Part print with two shaded views. Sizes in mm from the minimum x, y, z corner. A direction names the side the tool comes from. Give positions to 0.01 mm unless a question says otherwise; leave off trailing zeros. Loops run counter-clockwise (first coordinate to the right, second up) from the corner with the lowest first, then second, coordinate; pieces in that order, holes last. Notation, with made-up numbers: M 33.25,-31.5 L 90.25,-31.5 A38 cw 90.25,7.5 Z; hole C 0.5,68.25 d11. An arc over 180 degrees is marked long. Answer in a Markdown table with one row per item.
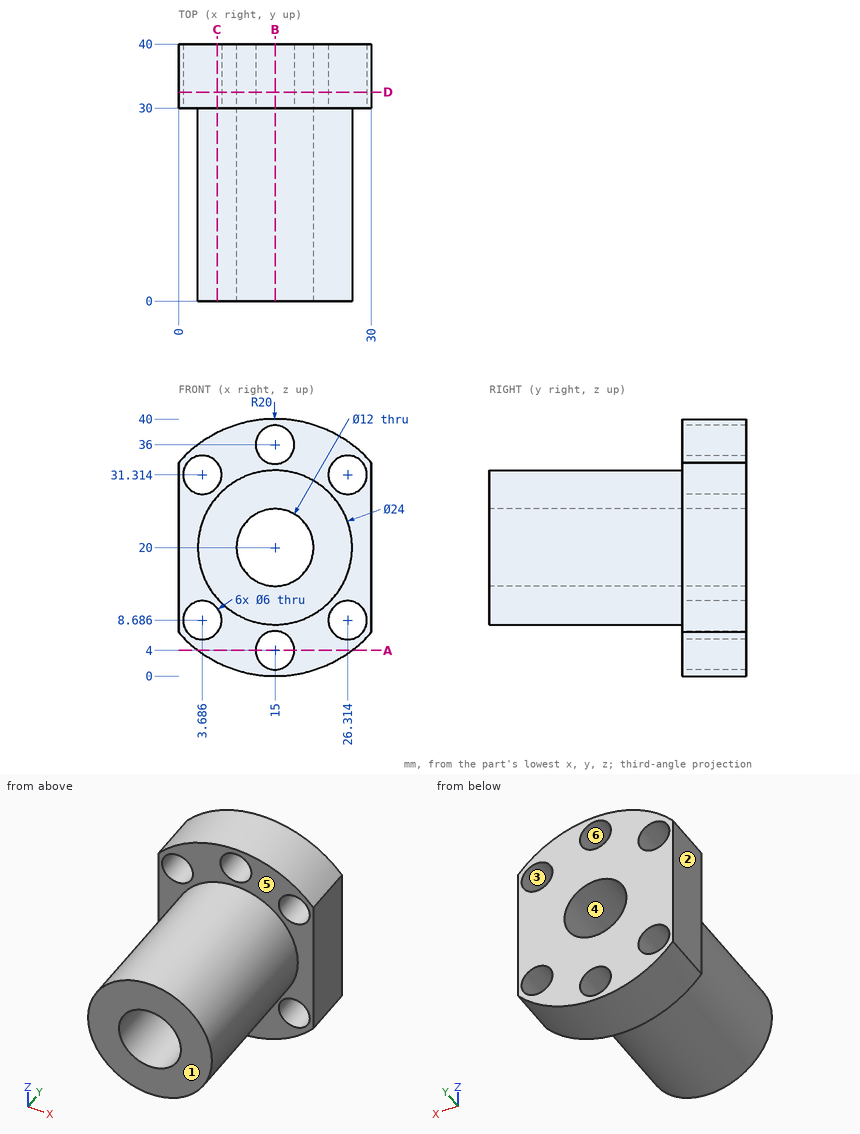
Q1. Drop flat-ended pins along their axis: pin 1 (1.5 mm diameter, centred on x = 18, y = 13, fed in from +Z); pin 2 (7 mm diameter, centred on x = 3.69, z = 8.69, fed in from -Y); pin 3 (2 mm diameter, centred on y = 19, z = 20.5, fed in from +X). Give the stop position or say it passes through.
Reported:
| item | result |
|---|---|
| pin 1 | z = 31.79 |
| pin 2 | y = 30 |
| pin 3 | x = 27 |
Q2. Mould opens along X. For the marked faces 1, 2, 3 and 4 say: released by +X, released by -X, zero draft, split by the parting line, or undercut.
Reported:
| item | result |
|---|---|
| face 1 | zero draft |
| face 2 | released by -X |
| face 3 | undercut |
| face 4 | undercut |
Q3. Saw through at C-C (x = 6). Give the cut face in (y, z).
Reported:
| item | result |
|---|---|
| outline | M 0,12.06 L 30,12.06 L 30,10.6 L 40,10.6 L 40,29.4 L 30,29.4 L 30,27.94 L 0,27.94 Z; M 30,2.14 L 40,2.14 L 40,6.78 L 30,6.78 Z; M 30,33.22 L 40,33.22 L 40,37.86 L 30,37.86 Z |
Q4. Saw through at B-B (x = 15). Give the cut face in (y, z).
Reported:
| item | result |
|---|---|
| outline | M 0,8 L 30,8 L 30,7 L 40,7 L 40,14 L 0,14 Z; M 0,26 L 40,26 L 40,33 L 30,33 L 30,32 L 0,32 Z; M 30,0 L 40,0 L 40,1 L 30,1 Z; M 30,39 L 40,39 L 40,40 L 30,40 Z |
Q5. Probe probe 1 along Z at (x, y) = (15, 33.5); probe 2 along Z at (x, y) = (28.5, 31.5) (1 decimal); probe 3 along Z at (x, y) = (24.5, 32) (1 decimal). List the from-to ranges inside material, lowest first.
Reported:
| item | result |
|---|---|
| probe 1 | 0 to 1, 7 to 14, 26 to 33, 39 to 40 |
| probe 2 | 5.2 to 6.6, 10.7 to 29.3, 33.4 to 34.8 |
| probe 3 | 2.4 to 6.3, 11.1 to 28.9, 33.7 to 37.6 |
Q6. Saw through at A-A (z = 4). Give the cut face in (x, y), and give its area (3 significant figures).
Reported:
| item | result |
|---|---|
| outline | M 3,30 L 12,30 L 12,40 L 3,40 Z; M 18,30 L 27,30 L 27,40 L 18,40 Z |
| area | 180 mm² |
Q7. 3-axis set-ups, long thin cutter, end or side, ignore diameter. For the marked faces 5 and 6: which of +Z, -Z, +X, -X, +Y, -Y reach the whole face in a straight line?
Reported:
| item | result |
|---|---|
| face 5 | -Y |
| face 6 | +Y, -Y |
Q8. Saw through at D-D (y = 32.5). Give the cut face in (x, z).
Reported:
| item | result |
|---|---|
| outline | M 0,6.77 A20 ccw 30,6.77 L 30,33.23 A20 ccw 0,33.23 Z; hole C 3.69,8.69 d6; hole C 3.69,31.31 d6; hole C 15,20 d12; hole C 15,4 d6; hole C 15,36 d6; hole C 26.31,8.69 d6; hole C 26.31,31.31 d6 |
